Here's the drawing with two shaded views (mm, measured from the low corner). I have some questions. A direction names the side the tool comes from. Coordinates: 2 decimals unless noted, no trailing zeros. Write each loop counter-clockwise with the first axis right and the second up, starting at its lowest first coordinate (ties: lowest second). Pieces come first, ordered by that corner, then holes. Notation, with made-up numbers: (-20, 86.25) -> (6, 86.25) arc R13 ccw to (6, 92.25) -> close; hole circle Ø9 at (17, -17). An arc over 180 degrees is marked (long way). Put each result on its own line as item: value. Start each with the question number.
Item 1: I need wall thicknesses on line 1 (Y direction, x = 10, z = 1) (1 decimal); line 2 (X direction, y = 17.5, z = 6.25) (1 decimal); line 3 (Y direction, x = 10.25, z = 3.25) (1 decimal). Which ranges of each line are inside material? Lowest first, please. Write a range as [from, to].
Item 2: If we mould it in two halves opening along Y, with no side actions, what happens to the marked faces 3, 4 and 5? For each: released by +Y, released by -Y, zero draft, split by the parting line, or undercut.
Item 3: For pin 1 (3 mm diameter, centred on y = 16.5, z = 4, fed in from -X); pin 2 (3 mm diameter, centred on x = 29, y = 16.5, fed in from -Z), each with a flat end and sliding along its axis, tell me the tip position at first contact or that it passes through.
Item 4: I want a section at B-B, the plane y = 16.5. List the corners of the cut face in (x, z) for me.
Item 5: I want a section at C-C, the plane x = 22. List the corners of the cut face in (y, z) for me.
Item 6: On a 3-axis mill with a long thin cutter (end or side, diameter ignored), from which of +Z, -Z, +X, -X, +Y, -Y can I reach the whole of each face in a straight line? I mean the marked faces 1 and 2. Say none if no direction works.
Item 7: I want a section at A-A, the plane z = 4. State how many separate pieces and enclosed holes the cut face has, then the cut area to 3 significant figures.
Item 8: I want a section at D-D, the plane x = 11. List the corners of the cut face in (y, z) for me.
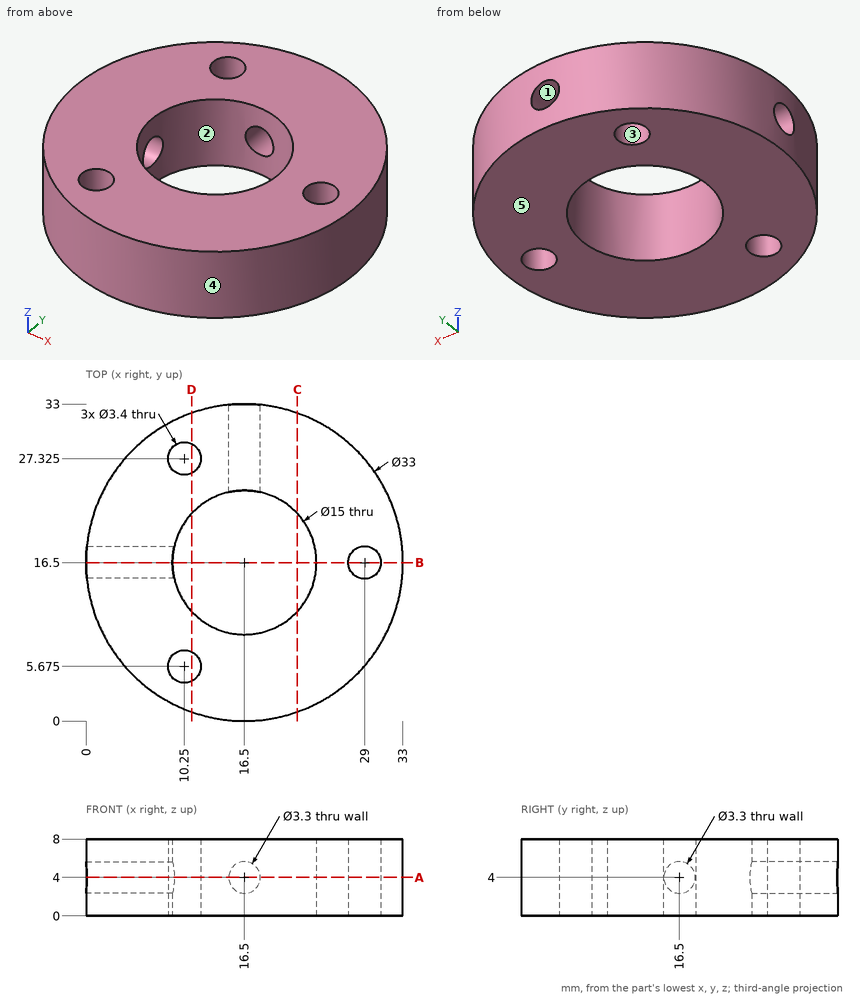
Calculated:
1. line 1: y = [1.3, 4], [7.4, 12.8], [20.2, 25.6], [29, 31.7]
1. line 2: x = [0, 9.1], [23.9, 27.6], [30.4, 33]
1. line 3: y = [1.2, 4], [7.4, 12.4], [20.6, 25.6], [29, 31.8]
2. face 3: undercut
2. face 4: split by the parting line
2. face 5: zero draft
3. pin 1: stops at x = 23.85
3. pin 2: passes through
4. outline: (0, 0) -> (9, 0) -> (9, 2.35) -> (0, 2.35) -> close; (0, 5.65) -> (9, 5.65) -> (9, 8) -> (0, 8) -> close; (24, 0) -> (27.3, 0) -> (27.3, 8) -> (24, 8) -> close; (30.7, 0) -> (33, 0) -> (33, 8) -> (30.7, 8) -> close
5. outline: (0.94, 0) -> (11.4, 0) -> (11.4, 8) -> (0.94, 8) -> close; (21.6, 0) -> (32.06, 0) -> (32.06, 8) -> (21.6, 8) -> close
6. face 1: +Y
6. face 2: +Z, -Z
7. separate pieces: 2
7. enclosed holes: 3
7. area: 592 mm2
8. outline: (0.94, 0) -> (4.15, 0) -> (4.15, 8) -> (0.94, 8) -> close; (7.2, 0) -> (11.4, 0) -> (11.4, 8) -> (7.2, 8) -> close; (21.6, 0) -> (25.8, 0) -> (25.8, 8) -> (21.6, 8) -> close; (28.85, 0) -> (32.06, 0) -> (32.06, 8) -> (28.85, 8) -> close
